Build history of the part. All positions in model axes, mm. A direction names the side the tool comes from. Round coordinates to 2 decimals unless told otherwise and drop trailing zeros. Write each loop counter-clockwise with the first axis right and the second up, starting at its lowest first coordinate (ties: lowest second). Pieces come first, ordered by that corner, then holes. Notation, with made-up numbers: (-29.5, 15.25) -> (-8.5, 15.25) arc R38 ccw to (-8.5, 54.25) -> close; hole circle Ø3 at (73, -1). An arc over 180 degrees is marked (long way). Answer in a Markdown table with one row per item.
```python
from build123d import *

# Parameters (mm, degrees)
F1_DEPTH = 3
F0_W     = 2.4358974359
F0_H     = 1.292
F0_W_2   = 8.6726998492
F0_H_2   = 1.1936711916
F0_W_3   = 7.094017094
F2_DEPTH = 6


with BuildPart() as f1:
    # F0 (on Top) → F1 (new body)
    with BuildSketch(Plane.XY):
        with BuildLine():
            Line((-19.5, -4.5), (-15, -4.5))
            Line((-15, -4.5), (-15, 0))
            Line((-15, 0), (-17.0055641305, 0))
            ThreePointArc((-17.0055641305, 0), (-19.5, -2.4944358695), (-21.9944358695, 0))
            Line((-21.9944358695, 0), (-24, 0))
            ThreePointArc((-24, 0), (-22.6819805153, -3.1819805153), (-19.5, -4.5))
        make_face()
        with BuildLine():
            Line((-17.0055641305, 0), (-15, 0))
            Line((-15, 0), (-15, 4.5))
            Line((-15, 4.5), (-19.5, 4.5))
            ThreePointArc((-19.5, 4.5), (-22.6819805153, 3.1819805153), (-24, 0))
            Line((-24, 0), (-21.9944358695, 0))
            ThreePointArc((-21.9944358695, 0), (-19.5, 2.4944358695), (-17.0055641305, 0))
        make_face()
        Polygon((-15, 0), (-15, -4.5), (-11.5585721468, -4.5), (-11.5585721468, 3.6675274007), (-14.6782302665, 3.6675274007), (-14.6782302665, 4.5), (-15, 4.5), align=None)
    extrude(amount=F1_DEPTH)



with BuildPart() as f1b:
    # F0 (on Top) → F1, piece 2 (new body)
    with BuildSketch(Plane.XY):
        Polygon((-9.1226747109, 3.6675274007), (-9.1226747109, -4.5), (-5.2295331336, -4.5), (-2.0654093324, 4.5), (-6.0055304173, 4.5), (-6.0055304173, 3.6675274007), align=None)
    extrude(amount=F1_DEPTH)


with BuildPart() as f1c:
    # F0 (on Top) → F1, piece 3 (new body)
    with BuildSketch(Plane.XY):
        Polygon((-2.2272498743, -3.056957265), (-2.6662637946, -4.5), (2.399798234, -4.5), (1.9607843137, -3.056957265), align=None)
    extrude(amount=F1_DEPTH)


with BuildPart() as f1d:
    # F0 (on Top) → F1, piece 4 (new body)
    with BuildSketch(Plane.XY):
        with BuildLine():
            Line((-1.6138763198, -1.0157305178), (1.3775766717, -1.0157305178))
            add(Edge.make_bspline(
                [(1.3775766717, -1.0157305178), (0.2237305178, 2.6997043741), (0.0779286073, 3.1873866264)],
                knots=[0, 0, 0, 1, 1, 1], degree=2))
            add(Edge.make_bspline(
                [(0.0779286073, 3.1873866264), (-0.0678733032, 3.6750688788), (-0.1307189542, 3.9566173957)],
                knots=[0, 0, 0, 1, 1, 1], degree=2))
            add(Edge.make_bspline(
                [(-0.1307189542, 3.9566173957), (-0.3896430367, 2.9510869784), (-1.6138763198, -1.0157305178)],
                knots=[0, 0, 0, 1, 1, 1], degree=2))
        make_face()
    extrude(amount=F1_DEPTH)


with BuildPart() as f1e:
    # F0 (on Top) → F1, piece 5 (new body)
    with BuildSketch(Plane.XY):
        Polygon((6.862745098, 4.5), (1.7854843124, 4.5), (4.9613779479, -4.5), (6.862745098, -4.5), align=None)
    extrude(amount=F1_DEPTH)


with BuildPart() as f1f:
    # F0 (on Top) → F1, piece 6 (new body)
    with BuildSketch(Plane.XY):
        Polygon((15, 4.5), (9.2986425339, 4.5), (9.2986425339, -3.7809391654), (13.9567621921, -3.7809391654), (13.9567621921, -4.5), (15, -4.5), align=None)
    extrude(amount=F1_DEPTH)


with BuildPart() as f1_1:
    add(f1.part)

    add(f1b.part)  # F2 merges F1b

    add(f1c.part)  # F2 merges F1c

    add(f1d.part)  # F2 merges F1d

    add(f1e.part)  # F2 merges F1e

    add(f1f.part)  # F2 merges F1f
    # F0 (on Top) → F2 (join)
    with BuildSketch(Plane.XY):
        Polygon((-11.5585721468, 3.6675274007), (-11.5585721468, -4.5), (-9.1226747109, -4.5), (-9.1226747109, 3.6675274007), (-6.0055304173, 3.6675274007), (-6.0055304173, 4.5), (-14.6782302665, 4.5), (-14.6782302665, 3.6675274007), align=None)
        with Locations((-10.3406234289, -5.146)):
            Rectangle(F0_W, F0_H)
        with Locations((-10.3418803419, 5.0968355958)):
            Rectangle(F0_W_2, F0_H_2)
        Polygon((-2.0654093324, 4.5), (-5.2295331336, -4.5), (-2.6662637946, -4.5), (-2.2272498743, -3.056957265), (1.9607843137, -3.056957265), (2.399798234, -4.5), (4.9613779479, -4.5), (1.7854843124, 4.5), align=None)
        with BuildLine():
            add(Edge.make_bspline(
                [(1.3775766717, -1.0157305178), (0.2237305178, 2.6997043741), (0.0779286073, 3.1873866264)],
                knots=[0, 0, 0, 1, 1, 1], degree=2))
            Line((1.3775766717, -1.0157305178), (-1.6138763198, -1.0157305178))
            add(Edge.make_bspline(
                [(-0.1307189542, 3.9566173957), (-0.3896430367, 2.9510869784), (-1.6138763198, -1.0157305178)],
                knots=[0, 0, 0, 1, 1, 1], degree=2))
            add(Edge.make_bspline(
                [(0.0779286073, 3.1873866264), (-0.0678733032, 3.6750688788), (-0.1307189542, 3.9566173957)],
                knots=[0, 0, 0, 1, 1, 1], degree=2))
        make_face(mode=Mode.SUBTRACT)
        Polygon((4.9613779479, -4.5), (2.399798234, -4.5), (2.792860734, -5.792), (5.4172951232, -5.792), align=None)
        Polygon((-2.6662637946, -4.5), (-5.2295331336, -4.5), (-5.6837606838, -5.792), (-3.0593262946, -5.792), align=None)
        Polygon((-1.628959276, 5.7414338864), (-2.0654093324, 4.5), (1.7854843124, 4.5), (1.3474107592, 5.7414338864), align=None)
        with Locations((10.409753645, -5.146)):
            Rectangle(F0_W_3, F0_H)
        Polygon((9.2986425339, 4.5), (6.862745098, 4.5), (6.862745098, -4.5), (13.9567621921, -4.5), (13.9567621921, -3.7809391654), (9.2986425339, -3.7809391654), align=None)
        with Locations((8.080693816, 5.0968355958)):
            Rectangle(F0_W, F0_H_2)
    extrude(amount=F2_DEPTH)


solid = f1_1.part
```
Q1. Wall check: line 1 (X direction, y = 0.5, z = 3.75); line 2 (Y direction, x = -19.5, z = 1.85); line 3 (X direction, y = -3.75, z = 5.75). Give the ranges that are in metal, low to high. Write a range as [from, to].
A:
| item | result |
|---|---|
| line 1 | [-11.56, -9.12], [-3.47, -1.15], [0.91, 3.2], [6.86, 9.3] |
| line 2 | [-4.5, -2.49], [2.49, 4.5] |
| line 3 | [-11.56, -9.12], [-4.97, -2.44], [2.17, 4.7], [6.86, 9.3] |
Q2. Which spindle directions (+Z, -Z, +X, -X, +Y, -Y) get a long thin tool onto all of the face, cutting with end or side? Do faces 4 (the flat face through (-13, 3.668, 4)), 5 (the flat face through (-17, 4.5, 1)), 6 (the flat face through (0, -1.016, 4)), 7 (the flat face through (14.5, -4.5, 1.5)). Say none if no direction does.
A:
| item | result |
|---|---|
| face 4 | +Z, -X, -Y |
| face 5 | +Z, -Z, -X, +Y |
| face 6 | +Z |
| face 7 | +Z, -Z, +X, -Y |
Q3. Saw through at B-B on x = 11. Write the cut outline in (y, z), plus the area to 3 significant figures.
A:
| item | result |
|---|---|
| outline | (-5.79, 0) -> (4.5, 0) -> (4.5, 3) -> (-3.78, 3) -> (-3.78, 6) -> (-5.79, 6) -> close |
| area | 36.9 mm² |
Q4. Drop flat-ended pins along their axis: P1, Ø3.5, axis at x = 0, z = 4.5, coming from the -Y side; P2, Ø5, axis at x = -12, y = 4, coming from the -Z side; P3, Ø1.2, axis at x = 0, y = -4, coming from the +Z side; P4, Ø1.5, axis at y = 1, z = 4.5, coming from the +X side. Give the stop position or say it passes through.
A:
| item | result |
|---|---|
| P1 | y = -4.5 |
| P2 | z = 0 |
| P3 | z = 3 |
| P4 | x = 9.3 |
Q5. Two-plate mould, pull along X, no slides. Class faces 1 (the flat face through (15, 0, 1)), 2 (the flat face through (0, -4.5, 1)), 3 (the flat face through (9, -1, 6)): released by +X, released by -X, zero draft, split by the parting line, or undercut.
A:
| item | result |
|---|---|
| face 1 | released by +X |
| face 2 | undercut |
| face 3 | zero draft |
Q6. Saw through at A-A on z = 3.5. State how many separate pieces and enclosed holes the cut face has, plus the area to 3 significant figures.
A:
| item | result |
|---|---|
| separate pieces | 3 |
| enclosed holes | 1 |
| area | 138 mm² |
